Work out the finished part from the listing and answer in its coordinate system (mm). A direction names the side the tool comes from. Round coordinates to 2 decimals unless told otherwise and drop trailing zeros. Order: outer loops, then holes, each group sorted by start corner. A loop starts at its lowest first (then second) coordinate and runs counter-clockwise, first axis right, second up. Notation, with made-up numbers: (-1, 50.5) - (21, 50.5) arc R16 cw to (21, 70.5) - close; hole circle Ø11 at (-14, -26.5). An arc over 180 degrees is marked (long way). Put each result on its own line as item: value.
```python
from build123d import *

# Parameters (mm, degrees)
PAD005_DEPTH           = 115
SKETCH004_W            = 115
SKETCH004_H            = 12
PAD004_DEPTH           = 190
FUSION_PLACEMENT_ANGLE = 180


with BuildPart() as body004:
    # CopySketch005 → Pad005 (new body)
    with BuildSketch(Plane.YZ):
        Polygon((-91, -17.296696), (20, 4.703304), (20, 16.703304), (-91, -11.296696), align=None)
    extrude(amount=PAD005_DEPTH)


with BuildPart() as fusion:
    # Sketch004 → Pad004 (new body)
    with BuildSketch(Plane.XZ):
        with Locations((57.5, -18.765628)):
            Rectangle(SKETCH004_W, SKETCH004_H)
    extrude(amount=PAD004_DEPTH)

    # Fusion: union Body004
    add(body004.part)


with BuildPart() as fusion_1:
    # Fusion placement: moved
    add(fusion.part.moved(Location((72, -332, 0))).rotate(Axis((72, -332, 0), (0, 0, 1)), FUSION_PLACEMENT_ANGLE))


solid = fusion_1.part
```
1) A cutting plane is placed at B-B on y = -312. Write down the section's boundary in (x, z), then the cut area to 3 significant figures.
Findings below:
outline: (-43, -24.77) - (72, -24.77) - (72, -12.77) - (-43, -12.77) - close; (-43, -3.22) - (72, -3.22) - (72, 6.61) - (-43, 6.61) - close
area: 2,510 mm2
2) Given pin 1 Ø5 at (x, y) = (-29.5, -274) entering from +Z; pin 2 Ø1.5 at (x, z) = (51, -17.5) entering from -Y; pin 3 Ø20.5 at (x, y) = (6.5, -304.5) entering from +Z; pin 4 Ø8 at (y, z) = (-254.5, -5) entering from -X, each flat-ended and moving along its own axis, determine where each tip first touches the part or whether it passes through.
Findings below:
pin 1: stops at z = -2.34
pin 2: stops at y = -332
pin 3: stops at z = 7.31
pin 4: stops at x = -43
3) For a pull along Z with two mould halves and no side action, classify faces 1 (the flat face through (15.305, -307.314, -4.153)), 2 (the flat face through (72, -248, -14)), 3 (the flat face through (15.3, -297.28, 2.9)) as pulls with the +Z half, pulls with the -Z half, needs draft (parallel to the pull), parting line crosses it, or undercut.
Findings below:
face 1: undercut
face 2: needs draft
face 3: pulls with the +Z half
4) For faces 4 (the flat face through (15, -352, 11)), 5 (the flat face through (15, -332, -19)), 6 (the flat face through (15, -192, -12.766)), determine the directions among +Z, -Z, +X, -X, +Y, -Y from which every point of the face is accessible in a straight line to the end or side of a thin tool.
Findings below:
face 4: +Z, -Z, +X, -X, -Y
face 5: -Z, +X, -X, -Y
face 6: +Z, +X, -X, +Y
5) Straight lines are drawn through the part: L1, parallel to Y at x = 61, z = -16; L2, parallel to Z at x = 34.5, y = -237; L3, parallel to Z at x = 57, y = -321. For each, find the intervals that lie inside material, in ascending order. Write a range as from..to.
Findings below:
L1: y = -332..-142
L2: z = -24.77..-12.77
L3: z = -24.77..-12.77, -1.44..8.88
6) A cutting plane is placed at C-C on y = -219.5. Write down the section's boundary in (x, z), then the cut area to 3 significant figures.
Findings below:
outline: (-43, -24.77) - (72, -24.77) - (72, -12.77) - (-43, -12.77) - close
area: 1,380 mm2
7) A cutting plane is placed at D-D on z = -18. Write down the section's boundary in (x, y), then the cut area to 4 significant figures.
Findings below:
outline: (-43, -332) - (72, -332) - (72, -142) - (-43, -142) - close
area: 21,850 mm2
8) A cutting plane is placed at A-A on x = -32. Write down the section's boundary in (y, z).
Findings below:
outline: (-352, 4.7) - (-263.86, -12.77) - (-332, -12.77) - (-332, -24.77) - (-142, -24.77) - (-142, -12.77) - (-241, -12.77) - (-241, -11.3) - (-352, 16.7) - close
